```python
from build123d import *

# Parameters (mm, degrees)
SKETCH1_R           = 4
BOSS_EXTRUDE1_DEPTH = 20


with BuildPart() as part:
    # Sketch1 → Boss-Extrude1 (new body)
    with BuildSketch(Plane(origin=(0, 0, 0), x_dir=(1, 0, 0), z_dir=(0, 1, 0))):
        with BuildLine():
            Line((30, -12.5), (-30, -12.5))
            Line((-30, -12.5), (-30, -6.90963498))
            Line((-30, -6.90963498), (-16, -6.90963498))
            ThreePointArc((-16, -6.90963498), (-11.757359313, -5.152275667), (-10, -0.90963498))
            Line((-10, -0.90963498), (-10, 0))
            ThreePointArc((-10, 0), (0, 10), (10, 0))
            Line((10, 0), (10, -0.90963498))
            ThreePointArc((10, -0.90963498), (11.757359313, -5.152275667), (16, -6.90963498))
            Line((16, -6.90963498), (30, -6.90963498))
            Line((30, -6.90963498), (30, -12.5))
        make_face()
        with Locations(Location((0, 0, 0), (0, 0, 270))):
            Circle(SKETCH1_R, mode=Mode.SUBTRACT)
    extrude(amount=BOSS_EXTRUDE1_DEPTH)


solid = part.part
```
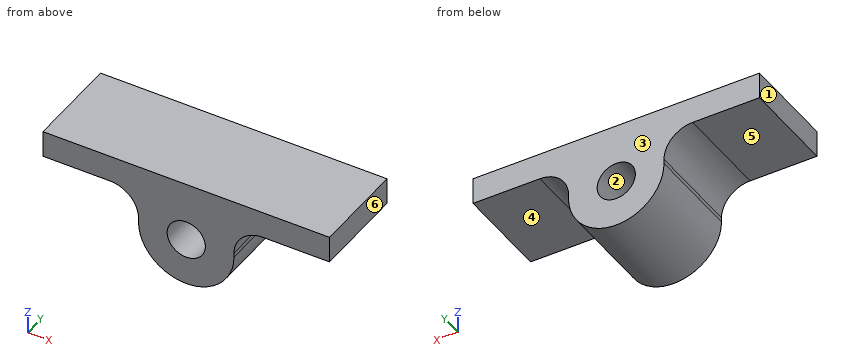
Could you check a few things on this model? Use its own coordinates, in mm. Face numbers are marked on the shaded views. A direction names the side the tool comes from. Coordinates: 2 decimals unless noted, no trailing zeros. Loops run counter-clockwise (first coordinate to the right, second up) from the corner with the lowest first, then second, coordinate; pieces in that order, holes last.
1) Please list where these lines run through material, in increasing order: line 1 along X through (y, z) = (15.5, 0); line 2 along Z through (x, y) = (3, 14.75); line 3 along Z through (x, y) = (25, 14).
Reported:
line 1: x = -10 to -4, 4 to 10
line 2: z = -9.54 to -2.65, 2.65 to 12.5
line 3: z = 6.91 to 12.5
2) Imagine slicing it at B-B (x = 0). List the corners of the cut face in (y, z) for me, and give its area (3 significant figures).
Reported:
outline: (0, -10) - (20, -10) - (20, -4) - (0, -4) - close; (0, 4) - (20, 4) - (20, 12.5) - (0, 12.5) - close
area: 290 mm2
3) Imagine slicing it at C-C (x = -8). List the corners of the cut face in (y, z) for me.
Reported:
outline: (0, -6) - (20, -6) - (20, 12.5) - (0, 12.5) - close
4) Imagine slicing it at D-D (x = 18). List the corners of the cut face in (y, z) for me, and give its area (3 significant figures).
Reported:
outline: (0, 6.91) - (20, 6.91) - (20, 12.5) - (0, 12.5) - close
area: 112 mm2
5) Thinking about a two-plate mould opening in X: for the marked faces 1, 2 and 3, which applies, released by +X, released by -X, zero draft, split by the parting line, or undercut?
Reported:
face 1: released by -X
face 2: undercut
face 3: zero draft
6) Which directions (+Z, -Z, +X, -X, +Y, -Y) give clear straight access to the entire face, cutting with the end or side of a thin tool? Please do the marked faces 4, 5 and 6.
Reported:
face 4: -Z, +X, +Y, -Y
face 5: -Z, -X, +Y, -Y
face 6: +Z, -Z, +X, +Y, -Y
7) Imagine slicing it at A-A (y = 16.75). List the corners of the cut face in (x, z) for me, and give its area (3 significant figures).
Reported:
outline: (-30, 6.91) - (-16, 6.91) arc R6 cw to (-10, 0.91) - (-10, 0) arc R10 ccw to (10, 0) - (10, 0.91) arc R6 cw to (16, 6.91) - (30, 6.91) - (30, 12.5) - (-30, 12.5) - close; hole circle Ø8 at (0, 0)
area: 596 mm2
8) Will these pins go through, and if not, where does the flat tip stop? pin 1 Ø8 at (x, z) = (20.5, 7.5) entering from -Y; pin 2 Ø10 at (x, y) = (18.5, 15.5) entering from -Z; pin 3 Ø1 at (y, z) = (15, -7) entering from -X; pin 4 Ø11 at (x, y) = (21.5, 13.5) entering from -Z.
Reported:
pin 1: stops at y = 0
pin 2: stops at z = 6.36
pin 3: stops at x = -7.6
pin 4: stops at z = 6.91
